```python
from build123d import *

# Parameters (mm, degrees)
SKETCH1_R                  = 4.9
BOSS_EXTRUDE1_DEPTH        = 2
SKETCH1_3_R                = 7.75
SKETCH1_3_R_2              = 4.9
BOSS_EXTRUDE2_DEPTH        = 6
BOSS_EXTRUDE3_START        = -3.8
SKETCH1_4_R                = 4.9
BOSS_EXTRUDE3_DEPTH        = 3.8
CSK_FOR_SFHCS1_D           = 3.2
CSK_FOR_SFHCS1_CSINK_D     = 6.72
CSK_FOR_SFHCS1_CSINK_ANGLE = 90
BOSS_EXTRUDE4_DEPTH        = 6
CIRPATTERN1_COUNT          = 6
CHAMFER2_SIZE              = 0.2
CHAMFER2_SIZE2             = 2
CHAMFER3_SIZE              = 0.1
CHAMFER3_SIZE2             = 2.5


with BuildPart() as part:
    # Sketch1 → Boss-Extrude1 (new body)
    with BuildSketch(Plane.XY):
        Circle(SKETCH1_R)
    extrude(amount=BOSS_EXTRUDE1_DEPTH)

    # Sketch1<3> → Boss-Extrude2 (add)
    with BuildSketch(Plane.XY):
        Circle(SKETCH1_3_R)
        Circle(SKETCH1_3_R_2, mode=Mode.SUBTRACT)
    extrude(amount=BOSS_EXTRUDE2_DEPTH)

    # Sketch1<4> → Boss-Extrude3 (add)
    with BuildSketch(Plane.XY.offset(BOSS_EXTRUDE3_START)):
        Circle(SKETCH1_4_R)
    extrude(amount=BOSS_EXTRUDE3_DEPTH)

    # CSK for  SFHCS1 (through all)
    with Locations(Plane.XY.offset(2)):
        with Locations((0, 0)):
            CounterSinkHole(CSK_FOR_SFHCS1_D / 2, CSK_FOR_SFHCS1_CSINK_D / 2, counter_sink_angle=CSK_FOR_SFHCS1_CSINK_ANGLE)

    # Sketch1<5> → Boss-Extrude4 (add)
    with BuildSketch(Plane.XY):
        with BuildLine():
            ThreePointArc((0.243261431, 4.842346934), (0.266872757, 4.878154286), (0.308005444, 4.890310077))
            ThreePointArc((0.308005444, 4.890310077), (1.2e-08, 4.9), (-0.308005421, 4.890310078))
            ThreePointArc((-0.308005421, 4.890310078), (-0.266872748, 4.878154279), (-0.243261431, 4.842346934))
            ThreePointArc((-0.243261431, 4.842346934), (0, 4.65), (0.243261431, 4.842346934))
        make_face()
    boss_extrude4 = extrude(amount=BOSS_EXTRUDE4_DEPTH)

    # CirPattern1: Boss-Extrude4 ×6 about axis
    cirpattern1_axis = Axis((0, 0, 0), (0, 0, 1))
    for i in range(1, CIRPATTERN1_COUNT):
        add(boss_extrude4.rotate(cirpattern1_axis, i * 360 / CIRPATTERN1_COUNT))

    # Chamfer2
    chamfer2_edges = [part.edges().sort_by_distance(p)[0] for p in [
        (-4.091169155, -2.670195719, 6),
        (-4.358041914, -2.207958555, 6),
        (-4.027018128, -2.325, 6),
        (2.44999999, -4.243524484, 6),
        (0.266872748, -4.878154279, 6),
        (-0.266872757, -4.878154286, 6),
        (0, -4.65, 6),
        (4.9, -1.2e-08, 6),
        (4.358041903, -2.20795856, 6),
        (4.091169156, -2.67019573, 6),
        (4.027018128, -2.325, 6),
        (2.45000001, 4.243524473, 6),
        (4.091169155, 2.670195719, 6),
        (4.358041914, 2.207958555, 6),
        (4.027018128, 2.325, 6),
        (-2.44999999, 4.243524484, 6),
        (-0.266872748, 4.878154279, 6),
        (0.266872757, 4.878154286, 6),
        (0, 4.65, 6),
        (-4.9, 1.2e-08, 6),
        (-4.358041903, 2.20795856, 6),
        (-4.091169156, 2.67019573, 6),
        (-4.027018128, 2.325, 6),
        (-2.45000001, -4.243524473, 6),
    ]]
    chamfer2_side = [part.faces().sort_by_distance(p)[0] for p in [
        (-7.530796898, 0, 6),
    ]]
    chamfer(chamfer2_edges, length=CHAMFER2_SIZE, length2=CHAMFER2_SIZE2, reference=chamfer2_side[0])

    # Chamfer3
    chamfer3_edges = [part.edges().sort_by_distance(p)[0] for p in [
        (-4.9, 0, -3.8),
    ]]
    chamfer3_side = [part.faces().sort_by_distance(p)[0] for p in [
        (-4.761407071, 0, -3.8),
    ]]
    chamfer(chamfer3_edges, length=CHAMFER3_SIZE, length2=CHAMFER3_SIZE2, reference=chamfer3_side[0])


solid = part.part
```
CAD build for the part. Positions are in the model's coordinates, mm. A direction names the side the tool comes from. Round coordinates to 2 decimals unless told otherwise and drop trailing zeros. Order: outer loops, then holes, each group sorted by start corner. A loop starts at its lowest first (then second) coordinate and runs counter-clockwise, first axis right, second up. Notation, with made-up numbers: (-6.5, 55.25) - (49.5, 55.25) arc R36 ccw to (49.5, 94.25) - close; hole circle Ø8 at (-37, 76.25). An arc over 180 degrees is marked (long way). Answer in a Markdown table with one row per item. Add a question column.
(1) Band-saw the part on A-A on y = 0. List the corners of the cut face in (x, z), and give its area (3 significant figures).
(2) Band-saw the part on B-B on z = 1.25. List the corners of the cut face in (x, y).
(3) Band-saw the part on D-D on x = -5.75. List the corners of the cut face in (y, z), and give its area (3 significant figures).
(4) 3-axis set-ups, long thin cutter, end or side, ignore diameter. For faces 1 (the face through (-2.477, -4.228, 2.986)), 2 (the face through (-1.062, -4.783, -0.659)), 3 (the face through (2, 0, -3.8)): which of +Z, -Z, +X, -X, +Y, -Y reach the whole face in a straight line?
(5) Probe L1, parallel to Y at x = 0, z = -1.35; L2, parallel to X at y = 0, z = -2.75. List the from-to ranges inside material, lowest first. Write a range as [from, to].
(6) Mould opens along Y. For faces 4 (the face through (-4.9, 0, 3)), 5 (the face through (2.477, 4.228, 2.986)), 6 (the face through (2.233, -4.294, -2.81)), 7 (the face through (-0.1, -5.1, 0)) say: +Y half, -Y half, draft (parallel to the pull), parting line (faces both ways), or undercut.
(7) Drop flat-ended pins along their axis: pin 1 Ø1.5 at (x, z) = (-1, -0.5) entering from -Y; pin 2 Ø2.5 at (x, y) = (0, 0) entering from +Z; pin 3 Ø4 at (y, z) = (3.5, 3) entering from +X. Give the stop position or say it passes through.
Data:
| question | item | result |
|---|---|---|
| 1 | outline | (-7.75, 0) - (-4.9, 0) - (-4.9, -1.3) - (-4.8, -3.8) - (-1.6, -3.8) - (-1.6, 0.24) - (-3.36, 2) - (-4.9, 2) - (-4.9, 4) - (-5.1, 6) - (-7.75, 6) - close; (1.6, -3.8) - (4.8, -3.8) - (4.9, -1.3) - (4.9, 0) - (7.75, 0) - (7.75, 6) - (5.1, 6) - (4.9, 4) - (4.9, 2) - (3.36, 2) - (1.6, 0.24) - close |
| 1 | area | 68.7 mm^2 |
| 2 | outline | circle Ø15.5 at (0, 0); hole circle Ø5.22 at (0, 0) |
| 3 | outline | (-5.2, 0) - (5.2, 0) - (5.2, 6) - (-5.2, 6) - close |
| 3 | area | 62.4 mm^2 |
| 4 | face 1 | +Z |
| 4 | face 2 | -Z |
| 4 | face 3 | -Z, +X, -X, +Y, -Y |
| 5 | L1 | y = [-4.9, -1.6], [1.6, 4.9] |
| 5 | L2 | x = [-4.84, -1.6], [1.6, 4.84] |
| 6 | face 4 | undercut |
| 6 | face 5 | undercut |
| 6 | face 6 | parting line |
| 6 | face 7 | draft |
| 7 | pin 1 | stops at y = -7.74 |
| 7 | pin 2 | passes through |
| 7 | pin 3 | stops at x = 7.6 |
